```python
from build123d import *

# Parameters (mm, degrees)
BOSS_EXTRUDE1_DEPTH = 63.5


with BuildPart() as part:
    # Sketch1 → Boss-Extrude1 (new body, symmetric)
    with BuildSketch(Plane(origin=(0, 57.843753362, -2.3797e-05), x_dir=(-1, 0, 0), z_dir=(0, -0.99999992, 0.0003994))):
        Polygon((-412.265833354, -477.954450626), (-183.665833354, -477.954450626), (-158.265833354, -452.554448601), (-158.265833354, -386.787080658), (-348.765833354, -386.787080658), (-348.765833354, 347.545615216), (489.434166646, 347.545615216), (489.434166646, -386.787080658), (298.934166646, -386.787080658), (298.934166646, -452.554448601), (324.334166646, -477.954450626), (552.934166646, -477.954450626), (578.334166646, -452.554448601), (578.334166646, 411.04562028), (552.934166646, 436.445622306), (-412.265833354, 436.445622306), (-437.665833354, 411.04562028), (-437.665833354, -452.554448601), align=None)
    extrude(amount=BOSS_EXTRUDE1_DEPTH, both=True)


solid = part.part
```
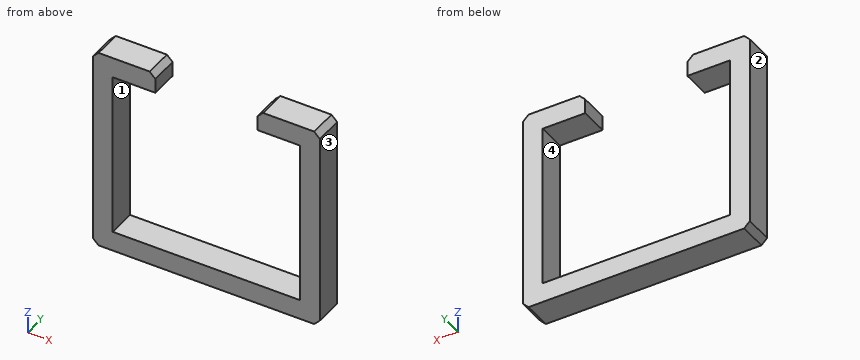
Check sheet for the modelled part. Datum: model origin and axes. Units: mm. Face numbers are marked on the shaded views. Round coordinates to 2 decimals unless told otherwise and drop trailing zeros. Order: outer loops, then holes, each group sorted by start corner. A loop starts at its lowest first (then second) coordinate and runs counter-clockwise, first axis right, second up.
1) Section check D-D (x = 127.5). Record the boundary of the cut face in (y, z).
2) Scan lines: line 1 (X direction, y = 99, z = 441); line 2 (X direction, y = 46, z = 16.5); line 3 (Z direction, x = -359, y = 55.5). Record each from-to range of solid material in increasing order.
3) Mould release check, pull along X, two halves, no side actions. Record for the marked faces 1, 2, 3 and 4: +X half, -X half, draft (parallel to the pull), parting line (faces both ways), or undercut.
4) Section check A-A (x = 255.5). Record the boundary of the cut face in (y, z).
5) Section check B-B (z = -102.5). Record the boundary of the cut face in (x, y).
6) Section check C-C (y = 36.5). Record the boundary of the cut face in (x, z).
Result:
1. outline: (-5.83, -436.42) - (121.17, -436.47) - (121.2, -347.57) - (-5.8, -347.52) - close
2. line 1: x = -578.33 to -298.93, 158.27 to 437.67
2. line 2: x = -578.33 to -489.43, 348.77 to 437.67
2. line 3: z = -436.44 to -347.54, 386.79 to 477.96
3. face 1: undercut
3. face 2: -X half
3. face 3: +X half
3. face 4: undercut
4. outline: (-5.83, -436.42) - (121.17, -436.47) - (121.2, -347.57) - (-5.8, -347.52) - close; (-5.5, 386.81) - (121.5, 386.76) - (121.53, 477.93) - (-5.47, 477.98) - close
5. outline: (-578.33, -5.7) - (-489.43, -5.7) - (-489.43, 121.3) - (-578.33, 121.3) - close; (348.77, -5.7) - (437.67, -5.7) - (437.67, 121.3) - (348.77, 121.3) - close
6. outline: (-578.33, -411.04) - (-552.93, -436.44) - (412.27, -436.44) - (437.67, -411.04) - (437.67, 452.56) - (412.27, 477.96) - (183.67, 477.96) - (158.27, 452.56) - (158.27, 386.8) - (348.77, 386.8) - (348.77, -347.54) - (-489.43, -347.54) - (-489.43, 386.8) - (-298.93, 386.8) - (-298.93, 452.56) - (-324.33, 477.96) - (-552.93, 477.96) - (-578.33, 452.56) - close
